Geometry: see drawing. Coordinates: mm, zero at the bounding-box minimum. Coordinates: 2 decimals unless noted, no trailing zeros. Write each loop counter-clockwise with the first axis right and the second up, starting at its lowest first coordinate (ties: lowest second). Pieces come first, ordered by that corner, then holes. Notation, with made-up numbers: M 44.5,78 L 50.5,78 A12 cw 50.5,86 Z; hole C -4,-25.5 d11. An arc over 180 degrees is marked long. Write item = value, one per line. Start each with the question number.
1. Pin query (flat end, axial travel): pin 1 Ø1.5 at (y, z) = (37.5, 2) entering from -X; pin 2 Ø1.5 at (y, z) = (23, 2) entering from -X. Return the tip coordinate at first contact, or that it passes through.
2. Line query: line 1 along Y through (x, z) = (80, 1.4); line 2 along X through (y, z) = (48, 1.95); line 3 along X through (y, z) = (19, 0.9). Output: solid intervals per line, ascending.
3. Section query A-A (x = 11.5). Output: boundary loops of the cut face in (y, z) (1 decimal).
4. Section query C-C (x = 67). Output: boundary loops of the cut face in (y, z), then the cut area to 3 significant figures.
5. Section query D-D (y = 7.5). Output: boundary loops of the cut face in (x, z).
6. Section query B-B (z = 1.95). Output: boundary loops of the cut face in (x, y).
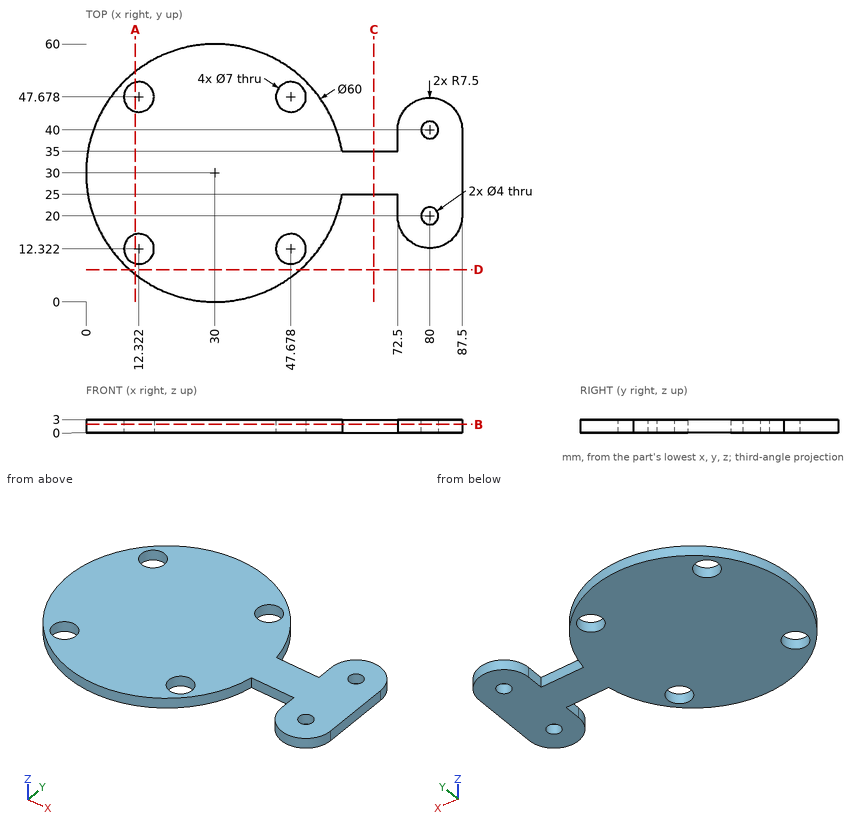
Results are:
q1.pin_1 = 0.77
q1.pin_2 = 0.66
q2.line_1 = 12.5 to 18, 22 to 38, 42 to 47.5
q2.line_2 = 6 to 8.84, 15.81 to 44.19, 51.16 to 54
q2.line_3 = 2.09 to 57.91, 72.57 to 78.27, 81.73 to 87.43
q3.outline = M 6.4,0 L 8.9,0 L 8.9,3 L 6.4,3 Z; M 15.7,0 L 44.3,0 L 44.3,3 L 15.7,3 Z; M 51.1,0 L 53.6,0 L 53.6,3 L 51.1,3 Z
q4.outline = M 25,0 L 35,0 L 35,3 L 25,3 Z
q4.area = 30.0 mm^2
q5.outline = M 10.16,0 L 49.84,0 L 49.84,3 L 10.16,3 Z
q6.outline = M 59.58,25 L 72.5,25 L 72.5,20 A7.5 ccw 87.5,20 L 87.5,40 A7.5 ccw 72.5,40 L 72.5,35 L 59.58,35 A30 ccw long Z; hole C 12.32,12.32 d7; hole C 12.32,47.68 d7; hole C 47.68,12.32 d7; hole C 47.68,47.68 d7; hole C 80,20 d4; hole C 80,40 d4
